Autodesk Inventor part; units mm, degrees
ref_plane "YZ Plane" through (0, 0, 0) normal (1, 0, 0) x (0, 1, 0)
ref_plane "XZ Plane" through (0, 0, 0) normal (0, 1, 0) x (-1, 0, 0)
ref_plane "XY Plane" through (0, 0, 0) normal (0, 0, 1) x (1, 0, 0)
sketch "Sketch1" plane through (0, 0, 0) normal (0, 1, 0) x (-1, 0, 0)
  circle A0 centre (0, 0) radius 14
  dimension "d0" = 28
extrude "Extrusion1" add sketch "Sketch1" along normal blind 24
chamfer "Chamfer1" distance 2 distance2 5 1 edges at (14, 0, 0) measured on face at (-0.5625, 0, 1.5565)
sketch "Sketch2" plane through (0, 0, 0) normal (0, -1, 0) x (1, 0, 0)
  circle A0 centre (0, 0) radius 9.5
  circle A1 centre (0, 0) radius 8
  line L0 (0, 0) -> (0, 9.5)
  line L1 (0, 0) -> (0, -9.5)
  line L2 (0, 0) -> (8, 0)
  line L3 (0, 0) -> (-8, 0)
  dimension "d6" = 19
  dimension "d7" = 16
hole "Hole1" at (0, 0, 9.5) at (-8, 0, 0) at (8, 0, 0) at (0, 0, -9.5) direction (0, 1, 0) diameter 3 depth 5 tip angle 118
chamfer "Chamfer2" distance 8 distance2 5 1 edges at (14, 24, 0) measured on face at (-0.5625, 24, 1.5565)
sketch "Sketch3" plane through (0, 24, 0) normal (0, 1, 0) x (1, 0, 0)
  circle A0 centre (0, 0) radius 1.5
  dimension "d18" = 3
extrude "Extrusion2" add sketch "Sketch3" along normal blind 4
sketch "Sketch4" plane through (0, 0, 0) normal (0, -1, 0) x (1, 0, 0)
  circle A0 centre (0, 0) radius 1.5
  dimension "d21" = 3
extrude "Extrusion3" add sketch "Sketch4" along normal blind 2
properties part number "motor_generic" material "Aluminum 6061"
For this review, take the finished solid that the model builds, in its own axes (mm). A direction names the side the tool comes from. Round coordinates to 2 decimals unless told otherwise and drop trailing zeros. Write each loop counter-clockwise with the first axis right and the second up, starting at its lowest first coordinate (ties: lowest second). Pieces come first, ordered by that corner, then holes. Notation, with made-up numbers: (-32.5, 65) - (-25.5, 65) arc R26 cw to (-25.5, 79) - close; hole circle Ø9 at (3, 34). An arc over 180 degrees is marked (long way). Answer as a JSON object with one key per item and string values.
1. Tool access review of faces 1 (the face through (0, 28, 0)), 2 (the face through (-6.536, 2.535, 0.325)), 3 (the face through (-1.2, 24, -1.2)): name each direction out of +Z, -Z, +X, -X, +Y, -Y from which nothing blocks a thin tool from reaching the whole face with its end or side.
Response values:
{"face 1": "+Z, -Z, +X, -X, +Y", "face 2": "-Y", "face 3": "+Y"}
2. For pin 1 Ø1.5 at (y, z) = (12.5, -1.5) entering from -X; pin 2 Ø6 at (x, z) = (8, 8) entering from -Y; pin 3 Ø1.8 at (x, z) = (0, -9.5) entering from +Y (3 decimals), all flat-tipped, find the tip position at first contact; note any pin that passes through.
Response values:
{"pin 1": "stops at x = -13.98", "pin 2": "stops at y = 0", "pin 3": "stops at y = 22.375"}
3. We need section A-A on y = 3.25. Give the boundary of the cut face in (x, z), then the cut area to 3 significant figures.
Response values:
{"outline": "circle Ø26.6 at (0, 0); hole circle Ø3 at (-8, 0); hole circle Ø3 at (0, -9.5); hole circle Ø3 at (0, 9.5); hole circle Ø3 at (8, 0)", "area": "527 mm2"}
4. We need section C-C on y = 10. Give the boundary of the cut face in (x, z).
Response values:
{"outline": "circle Ø28 at (0, 0)"}
5. We need section B-B on y = 22. Give the boundary of the cut face in (x, z), then the cut area to 3 significant figures.
Response values:
{"outline": "circle Ø18.4 at (0, 0)", "area": "266 mm2"}
6. Draft analysis for pull direction Z (two halves, no side actions). For faces 4 (the face through (0, 3, 11)), 5 (the face through (0, -2, 0)), 6 (the face through (-1.5, -0.99, -0.07)), state which applies: +Z half, -Z half, draft (parallel to the pull), parting line (faces both ways), or undercut.
Response values:
{"face 4": "undercut", "face 5": "draft", "face 6": "parting line"}
7. To check wall thickness, follow line 1 along X through (y, z) = (3.6, 0); line 2 along X through (y, z) = (3.35, 0); line 3 along Z through (x, y) = (0, 3.3). State the ranges of each line that lie inside material, in increasing order.
Response values:
{"line 1": "x = -13.44 to -9.5, -6.5 to 6.5, 9.5 to 13.44", "line 2": "x = -13.34 to -9.5, -6.5 to 6.5, 9.5 to 13.34", "line 3": "z = -13.32 to -11, -8 to 8, 11 to 13.32"}
